from build123d import *

# Parameters (mm, degrees)
SKETCH1_W           = 15
SKETCH1_H           = 10
SKETCH1_H_2         = 78
BOSS_EXTRUDE1_DEPTH = 5
SKETCH1_3_W         = 15
SKETCH1_3_H         = 10
BOSS_EXTRUDE2_DEPTH = 15
HOLE1_D             = 1
HOLE1_CBORE_D       = 8
HOLE1_CBORE_DEPTH   = 3
SKETCH1_4_W         = 15
SKETCH1_4_H         = 10
BOSS_EXTRUDE3_DEPTH = 87
HOLE2_START         = 41
HOLE2_OUTLINE_R     = 4
HOLE2_DEPTH         = 8
HOLE2_START_2       = 39
HOLE2_2_OUTLINE_R   = 0.5
HOLE2_2_DEPTH       = 2
CUT_EXTRUDE1_REACH  = 125.973
SKETCH9_R           = 3
CHAMFER1_SIZE       = 2.5
CHAMFER2_SIZE       = 1
CHAMFER3_SIZE       = 1


# Read off the part's stored shape, not the designer's step: Hole2
with BuildPart() as part:
    # Sketch1 → Boss-Extrude1 (new body)
    with BuildSketch(Plane.XY):
        with Locations((0, -44)):
            Rectangle(SKETCH1_W, SKETCH1_H)
        Rectangle(SKETCH1_W, SKETCH1_H_2)
        with Locations((0, 44)):
            Rectangle(SKETCH1_W, SKETCH1_H)
    extrude(amount=BOSS_EXTRUDE1_DEPTH)

    # Sketch1<3> → Boss-Extrude2 (add)
    with BuildSketch(Plane.XY):
        with Locations((0, -44)):
            Rectangle(SKETCH1_3_W, SKETCH1_3_H)
        with Locations((0, 44)):
            Rectangle(SKETCH1_3_W, SKETCH1_3_H)
    extrude(amount=-BOSS_EXTRUDE2_DEPTH)

    # Hole1 (through all)
    with Locations(Plane.XY.offset(5)):
        with Locations((0, 24.5), (0, 12.25), (0, 0), (0, -12.25), (0, -24.5)):
            CounterBoreHole(HOLE1_D / 2, HOLE1_CBORE_D / 2, HOLE1_CBORE_DEPTH)

    # Sketch1<4> → Boss-Extrude3 (add)
    with BuildSketch(Plane.XY):
        with Locations((0, -44)):
            Rectangle(SKETCH1_4_W, SKETCH1_4_H)
    extrude(amount=BOSS_EXTRUDE3_DEPTH)

    # Hole2 outline → Hole2 (cut)
    with BuildSketch(Plane(origin=(0, 0, 0), x_dir=(1, 0, 0), z_dir=(0, 1, 0)).offset(HOLE2_START)):
        with Locations((0, 7.5)):
            Circle(HOLE2_OUTLINE_R)
    extrude(amount=HOLE2_DEPTH, mode=Mode.SUBTRACT)

    # Hole2 2 outline → Hole2 2 (cut)
    with BuildSketch(Plane(origin=(0, 0, 0), x_dir=(1, 0, 0), z_dir=(0, 1, 0)).offset(HOLE2_START_2)):
        with Locations((0, 7.5)):
            Circle(HOLE2_2_OUTLINE_R)
    extrude(amount=HOLE2_2_DEPTH, mode=Mode.SUBTRACT)

    # Sketch9 → Cut-Extrude1 (cut, up to next)
    with BuildSketch(Plane(origin=(0, -39, 0), x_dir=(1, 0, 0), z_dir=(0, 1, 0)), mode=Mode.PRIVATE) as cut_extrude1_sk1:
        with Locations(Location((0, -27, 0), (0, 0, 270))):
            Circle(SKETCH9_R)
    cut_extrude1_tool1 = extrude(cut_extrude1_sk1.sketch, amount=-CUT_EXTRUDE1_REACH, mode=Mode.PRIVATE) & part.part
    # Sketch9 → Cut-Extrude1 (cut, up to next)
    with BuildSketch(Plane(origin=(0, -39, 0), x_dir=(1, 0, 0), z_dir=(0, 1, 0)), mode=Mode.PRIVATE) as cut_extrude1_sk2:
        with Locations(Location((0, -79.5, 0), (0, 0, 270))):
            Circle(SKETCH9_R)
    cut_extrude1_tool2 = extrude(cut_extrude1_sk2.sketch, amount=-CUT_EXTRUDE1_REACH, mode=Mode.PRIVATE) & part.part
    add(cut_extrude1_tool1.solids().sort_by_distance((0, -39, 27))[0], mode=Mode.SUBTRACT)
    add(cut_extrude1_tool2.solids().sort_by_distance((0, -39, 79.5))[0], mode=Mode.SUBTRACT)

    # Chamfer1
    chamfer1_edges = [part.edges().sort_by_distance(p)[0] for p in [
        (-4, 49, -7.5),
    ]]
    chamfer(chamfer1_edges, length=CHAMFER1_SIZE)

    # Chamfer2
    chamfer2_edges = [part.edges().sort_by_distance(p)[0] for p in [
        (0, -39, 76.5),
        (0, -39, 24),
        (-4, -24.5, 5),
        (-4, -12.25, 5),
        (-4, 0, 5),
        (-4, 12.25, 5),
        (-4, 24.5, 5),
    ]]
    chamfer(chamfer2_edges, length=CHAMFER2_SIZE)

    # Chamfer3
    chamfer3_edges = [part.edges().sort_by_distance(p)[0] for p in [
        (7.5, -49, 36),
        (-7.5, -39, 46),
        (-7.5, -44, 87),
        (-7.5, -49, 36),
        (-7.5, 49, -5),
        (7.5, 49, -5),
        (-7.5, 5, 5),
        (7.5, -39, -7.5),
        (-7.5, -44, -15),
        (-7.5, -39, -7.5),
        (7.5, -44, -15),
        (-7.5, 0, 0),
        (7.5, 0, 0),
        (7.5, 39, -7.5),
        (-7.5, 39, -7.5),
        (7.5, 44, -15),
        (-7.5, 44, -15),
        (7.5, 5, 5),
        (7.5, -44, 87),
        (7.5, -39, 46),
    ]]
    chamfer(chamfer3_edges, length=CHAMFER3_SIZE - 0.0001)  # a hair under: the kernel refuses the full size


solid = part.part
The listing builds one solid part. Answer for the finished solid, in the listing's coordinates (mm). A direction names the side the tool comes from. Give positions to 0.01 mm unless a question says otherwise; leave off trailing zeros. Write each loop counter-clockwise with the first axis right and the second up, starting at its lowest first coordinate (ties: lowest second). Pieces come first, ordered by that corner, then holes. Notation, with made-up numbers: (16, -19.75) -> (67, -19.75) arc R26 ccw to (67, 19.25) -> close; hole circle Ø1 at (34, -30). An arc over 180 degrees is marked (long way). One line per question, with ' | ' between items. Start each with the question number.
1. Section C-C (x = 1.75) is taken. State how many separate pieces and enclosed holes the cut face has, plus the area to 3 significant figures.
2. Section B-B (z = 48) is taken. Determine the outline of the cut face in (x, y).
3. For faces 1 (the flat face through (0, 44, -15)), 2 (the cylindrical face through (0, -44, 24)), 3 (the cylindrical face through (-0.867, 43.712, -3.595)), 4 (the flat face through (0, -39, 45)), 5 (the cylindrical face through (-0.867, -3.905, 3.014)), determine the directions among +Z, -Z, +X, -X, +Y, -Y from which every point of the face is accessible in a straight line to the end or side of a thin tool.
4. Section A-A (z = 79.5) is taken. Determine the outline of the cut face in (x, y).
5. For a pull along X with two mould halves and no side action, classify faces 6 (the flat face through (0, 11, 2)), 7 (the flat face through (7.5, -22, 3)), 8 (the flat face through (0, -44, 87)) as pulls with the +X half, pulls with the -X half, needs draft (parallel to the pull), parting line crosses it, or undercut.
6. Find the intervals of material crossed by probe 1 along Y at (x, z) = (0, 3.05); probe 2 along Y at (x, z) = (-3.75, -2); probe 3 along Z at (x, y) = (0.25, 45.5), in increasing order.
7. Given pin 1 Ø2.5 at (x, y) = (-0.5, 14) entering from +Z; pin 2 Ø9 at (x, z) = (0, -7.5) entering from +Y; pin 3 Ø9 at (x, y) = (0, 12.25) entering from +Z, each flat-ended and moving along its own axis, determine where each tip first touches the part or whether it passes through.
Response values:
1) separate pieces: 3 | enclosed holes: 0 | area: 1,330 mm2
2) outline: (-7.5, -48) -> (-6.5, -49) -> (6.5, -49) -> (7.5, -48) -> (7.5, -40) -> (6.5, -39) -> (-6.5, -39) -> (-7.5, -40) -> close
3) face 1: -Z, +X, -X, +Y, -Y | face 2: +Y, -Y | face 3: +Y | face 4: +Z, +X, -X, +Y | face 5: +Z
4) outline: (-7.5, -48) -> (-6.5, -49) -> (-3, -49) -> (-3, -40) -> (-4, -39) -> (-6.5, -39) -> (-7.5, -40) -> close; (3, -49) -> (6.5, -49) -> (7.5, -48) -> (7.5, -40) -> (6.5, -39) -> (4, -39) -> (3, -40) -> close
5) face 6: undercut | face 7: pulls with the +X half | face 8: needs draft
6) probe 1: -49 to -28.5, -20.5 to -16.25, -8.25 to -4, 4 to 8.25, 16.25 to 20.5, 28.5 to 49 | probe 2: -49 to -39, 39 to 49 | probe 3: -15 to -11.49, -3.51 to 5
7) pin 1: z = 2 | pin 2: y = 47 | pin 3: z = 4.5
